Study the drawing (mm; zero at the part's minimum x, y, z) and answer. Give positions to 0.01 mm unless a question says otherwise; leave off trailing zeros. Order: outer loops, then holes, each group sorted by start corner. A loop starts at its lowest first (then second) coordinate and runs counter-clockwise, first axis right, second up.
Item 1: A cutting plane is placed at A-A (x = 19.05). Write down the section's boundary in (y, z), plus the area to 3 significant figures.
Item 2: A cutting plane is placed at B-B (y = 18.25). Write down the section's boundary in (x, z) (3 decimals), plus the area to 3 significant figures.
Item 3: Find the intervals of material crossed by line 1 along Y through (x, z) = (19.05, 3.6); line 2 along Y through (x, z) = (68.25, 2.3); line 3 along Y through (x, z) = (62, 2.9), in increasing order.
Item 4: Given pin 1 Ø3 at (x, y) = (47.65, 18.25) entering from +Z; pin 2 Ø1 at (y, z) = (10.5, 0.5) entering from +X, each flat-ended and moving along its own axis, determine where each tip first touches the part or whether it passes through.
Item 5: A cutting plane is placed at C-C (z = 2.55). Write down the section's boundary in (x, y) (3 decimals), plus the area to 3 significant figures.
Item 6: A cutting plane is placed at D-D (x = 47.65). Write down the section's boundary in (y, z), plus the area to 3 significant figures.
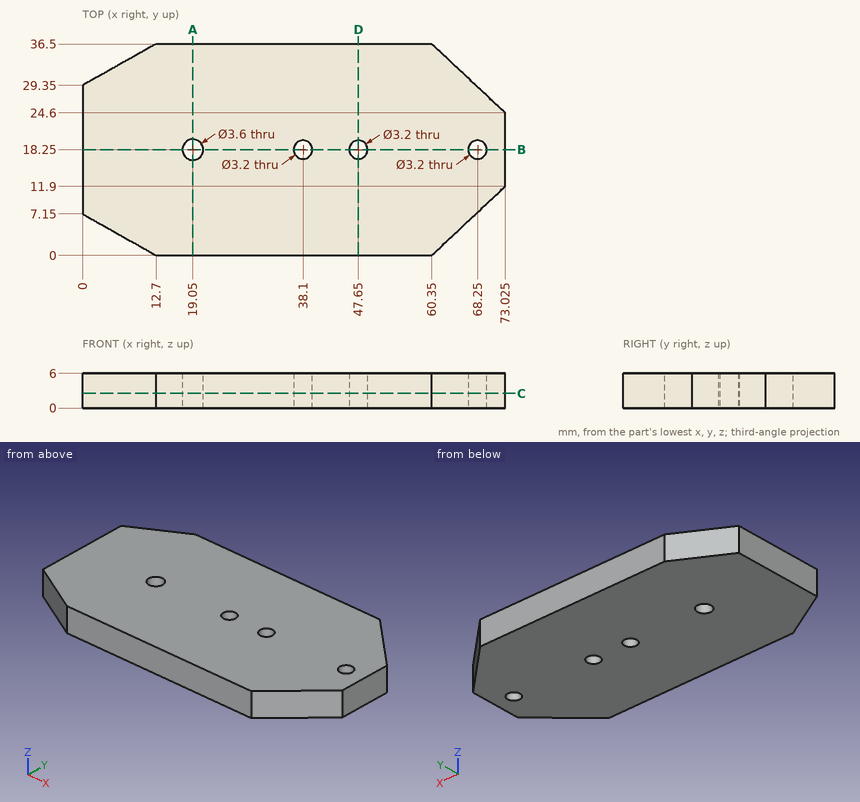
Response values:
1. outline: (0, 0) - (16.45, 0) - (16.45, 6) - (0, 6) - close; (20.05, 0) - (36.5, 0) - (36.5, 6) - (20.05, 6) - close
1. area: 197 mm2
2. outline: (0, 0) - (17.25, 0) - (17.25, 6) - (0, 6) - close; (20.85, 0) - (36.5, 0) - (36.5, 6) - (20.85, 6) - close; (39.7, 0) - (46.05, 0) - (46.05, 6) - (39.7, 6) - close; (49.25, 0) - (66.65, 0) - (66.65, 6) - (49.25, 6) - close; (69.85, 0) - (73.025, 0) - (73.025, 6) - (69.85, 6) - close
2. area: 359 mm2
3. line 1: y = 0 to 16.45, 20.05 to 36.5
3. line 2: y = 7.42 to 16.65, 19.85 to 29.08
3. line 3: y = 1.55 to 34.95
4. pin 1: passes through
4. pin 2: stops at x = 72.07
5. outline: (0, 7.15) - (12.7, 0) - (60.35, 0) - (73.025, 11.9) - (73.025, 24.6) - (60.35, 36.5) - (12.7, 36.5) - (0, 29.35) - close; hole circle Ø3.6 at (19.05, 18.25); hole circle Ø3.2 at (38.1, 18.25); hole circle Ø3.2 at (47.65, 18.25); hole circle Ø3.2 at (68.25, 18.25)
5. area: 2,390 mm2
6. outline: (0, 0) - (16.65, 0) - (16.65, 6) - (0, 6) - close; (19.85, 0) - (36.5, 0) - (36.5, 6) - (19.85, 6) - close
6. area: 200 mm2
